```python
from build123d import *

# Parameters (mm, degrees)
F0_R     = 3.175
F1_DEPTH = 12.7
F2_W     = 6.35
F2_H     = 23.4397758459
F3_DEPTH = 25.4
F4_R     = 3.175
F6_DEPTH = 6.35
F5_R     = 3.175
F7_DEPTH = 6.35


with BuildPart() as f1:
    # F0 (on Front) → F1 (new body)
    with BuildSketch(Plane.XZ):
        Polygon((-11.0584168369, 42.5397964036), (-28.1292907894, 64.142785233), (-45.2001647418, 42.5397964036), (-45.2001647418, -46.9452900396), (-11.0584168369, -46.9452900396), align=None)
        with Locations((-28.1292907894, 51.1445705025)):
            Circle(F0_R, mode=Mode.SUBTRACT)
    extrude(amount=F1_DEPTH)

    # F2 (on face) → F3 (cut)
    with BuildSketch(Plane(origin=(13.886044542, 0, 10.9728759269), x_dir=(0, 1, 0), z_dir=(0.7846021358, 0, 0.6199995875))):
        with Locations((-6.35, 56.046827053)):
            Rectangle(F2_W, F2_H)
    extrude(amount=-F3_DEPTH, mode=Mode.SUBTRACT)

    # F4 (on face) → F6 (join)
    with BuildSketch(Plane(origin=(0, 0, 0), x_dir=(-1, 0, 0), z_dir=(0, 1, 0))):
        with Locations((28.1292907894, -40.5952900396)):
            Circle(F4_R)
    extrude(amount=F6_DEPTH)

    # F5 (on face) → F7 (join)
    with BuildSketch(Plane.XZ.offset(12.7)):
        with Locations((-28.1292907894, -40.5952900396)):
            Circle(F5_R)
    extrude(amount=F7_DEPTH)


solid = f1.part
```
Could you check a few things on this model? Use its own coordinates, in mm. A direction names the side the tool comes from. Round coordinates to 2 decimals unless told otherwise and drop trailing zeros. Write each loop counter-clockwise with the first axis right and the second up, starting at its lowest first coordinate (ties: lowest second). Pieces come first, ordered by that corner, then holes. Notation, with made-up numbers: M 47.25,-15.5 L 84.25,-15.5 A7 ccw 84.25,-5.5 Z; hole C -5.75,79 d11. An arc over 180 degrees is marked long. Answer in a Markdown table with one row per item. Add a question column.
Q1. If we mould it in two halves opening along X, with no side actions, what happens to faces 1 (the cylindrical face through (-26.66, -1.57, 48.33)), 2 (the flat face through (-28, -12.7, 9)), 3 (the flat face through (-36.545, -2.028, 53.493)), 4 (the flat face through (-23.42, -6.39, 37.99))? For each: +X half, -X half, draft (parallel to the pull), parting line (faces both ways), or undercut.
Q2. Imagine slicing it at B-B (y = -5). Please give me the cut outline in (x, z).
Q3. Imagine slicing it at A-A (x = -26). Please give me the cut outline in (y, z) (3 decimals).
Q4. On a 3-axis mill with a long thin cutter (end or side, diameter ignored), from which of +Z, -Z, +X, -X, +Y, -Y can I reach the whole of each face in a straight line? I mean faces 5 (the cylindrical face through (-27.441, 3.131, -43.695)), 6 (the cylindrical face through (-26.66, -11.09, 48.33)), 7 (the flat face through (-29, -9.525, 45)), 8 (the flat face through (-28, -19.05, -41)), 9 (the cylindrical face through (-25.196, -15.831, -41.811)). Say none if no direction works.
Q5. If I drill on line 1 (Y direction, x = -23, z = -31.5); line 2 (Z direction, x = -31, y = -0.5); line 3 (X direction, y = -7, z = 34), over which ranges is the centre line in solid material (lowest first)? Write a range as from..to.
Q6. Imagine slicing it at D-D (x = -19). Please give me the cut outline in (y, z) (3 decimals), then the cut area to 3 significant figures.
Q7. Will these pins go through, and if not, where does the flat tip stop? pin 1 Ø8.5 at (x, z) = (-28.13, 51.14) entering from -Y; pin 2 Ø1 at (x, y) = (-17.5, -12.5) entering from +Z; pin 3 Ø17 at (x, z) = (-34, 9) entering from +Y.
Q8. Imagine slicing it at C-C (z = 38). Please give me the cut outline in (x, y) (3 decimals).
Values:
| question | item | result |
|---|---|---|
| 1 | face 1 | undercut |
| 1 | face 2 | draft |
| 1 | face 3 | -X half |
| 1 | face 4 | undercut |
| 2 | outline | M -45.2,-46.95 L -11.06,-46.95 L -11.06,42.54 L -13.6,45.75 L -33.53,30 L -44.32,43.66 L -45.2,42.54 Z |
| 3 | outline | M -19.05,-42.95 L -12.7,-42.95 L -12.7,-46.945 L 0,-46.945 L 0,-42.95 L 6.35,-42.95 L 6.35,-38.24 L 0,-38.24 L 0,48.789 L -3.175,48.789 L -3.175,35.951 L -9.525,35.951 L -9.525,48.789 L -12.7,48.789 L -12.7,-38.24 L -19.05,-38.24 Z; M -12.7,53.5 L -9.525,53.5 L -9.525,61.448 L -12.7,61.448 Z; M -3.175,53.5 L 0,53.5 L 0,61.448 L -3.175,61.448 Z |
| 4 | face 5 | +Y |
| 4 | face 6 | +Y, -Y |
| 4 | face 7 | +Z |
| 4 | face 8 | +Z, -Z, +X, -X, -Y |
| 4 | face 9 | -Y |
| 5 | line 1 | -12.7..0 |
| 5 | line 2 | -46.95..49.79, 52.5..60.51 |
| 5 | line 3 | -45.2..-36.68, -28.47..-11.06 |
| 6 | outline | M -12.7,-46.945 L 0,-46.945 L 0,52.59 L -3.175,52.59 L -3.175,41.482 L -9.525,41.482 L -9.525,52.59 L -12.7,52.59 Z |
| 6 | area | 1,190 mm^2 |
| 7 | pin 1 | y = -12.7 |
| 7 | pin 2 | z = 51.32 |
| 7 | pin 3 | y = 0 |
| 8 | outline | M -45.2,-12.7 L -11.058,-12.7 L -11.058,0 L -45.2,0 Z; hole M -39.844,-9.525 L -23.407,-9.525 L -23.407,-3.175 L -39.844,-3.175 Z |
